Design review of the part built by this model. Coordinates are the model's own, in mm. Face numbers are marked on the shaded views. Coordinates: 2 decimals unless noted, no trailing zeros. Loops run counter-clockwise (first coordinate to the right, second up) from the corner with the lowest first, then second, coordinate; pieces in that order, holes last. Notation, with made-up numbers: M 71.25,78.25 L 118.25,78.25 A15 cw 118.25,98.25 Z; hole C 51,-27 d10. An arc over 180 degrees is marked long. Answer as CSV lines item,"result". Start each with the question number.
from build123d import *

# Parameters (mm, degrees)
F1_DEPTH = 100
F2_R     = 2
F2_R_2   = 1
F3_DEPTH = 14.501


with BuildPart() as f1:
    # F0 (on Right) → F1 (new body)
    with BuildSketch(Plane.YZ):
        with BuildLine():
            ThreePointArc((10, 8.5), (9.56066, 9.56066), (8.5, 10))
            Line((8.5, 10), (3, 10))
            Line((3, 10), (3, 8.5))
            Line((3, 8.5), (6, 8.5))
            Line((6, 8.5), (6, 7))
            Line((6, 7), (3.75, 4.5))
            Line((3.75, 4.5), (0, 4.5))
            Line((0, 4.5), (-3.75, 4.5))
            Line((-3.75, 4.5), (-6, 7))
            Line((-6, 7), (-6, 8.5))
            Line((-6, 8.5), (-3, 8.5))
            Line((-3, 8.5), (-3, 10))
            Line((-3, 10), (-8.5, 10))
            ThreePointArc((-8.5, 10), (-9.56066, 9.56066), (-10, 8.5))
            Line((-10, 8.5), (-10, 3))
            Line((-10, 3), (-8.5, 3))
            Line((-8.5, 3), (-8.5, 6))
            Line((-8.5, 6), (-7, 6))
            Line((-7, 6), (-4.5, 3.75))
            Line((-4.5, 3.75), (-4.5, 0))
            Line((-4.5, 0), (-4.5, -3.75))
            Line((-4.5, -3.75), (-7, -6))
            Line((-7, -6), (-8.5, -6))
            Line((-8.5, -6), (-8.5, -3))
            Line((-8.5, -3), (-10, -3))
            Line((-10, -3), (-10, -8.5))
            ThreePointArc((-10, -8.5), (-9.56066, -9.56066), (-8.5, -10))
            Line((-8.5, -10), (-3, -10))
            Line((-3, -10), (-3, -8.5))
            Line((-3, -8.5), (-6, -8.5))
            Line((-6, -8.5), (-6, -7))
            Line((-6, -7), (-3.75, -4.5))
            Line((-3.75, -4.5), (0, -4.5))
            Line((0, -4.5), (3.75, -4.5))
            Line((3.75, -4.5), (6, -7))
            Line((6, -7), (6, -8.5))
            Line((6, -8.5), (3, -8.5))
            Line((3, -8.5), (3, -10))
            Line((3, -10), (8.5, -10))
            ThreePointArc((8.5, -10), (9.56066, -9.56066), (10, -8.5))
            Line((10, -8.5), (10, -3))
            Line((10, -3), (8.5, -3))
            Line((8.5, -3), (8.5, -6))
            Line((8.5, -6), (7, -6))
            Line((7, -6), (4.5, -3.75))
            Line((4.5, -3.75), (4.5, 0))
            Line((4.5, 0), (4.5, 3.75))
            Line((4.5, 3.75), (7, 6))
            Line((7, 6), (8.5, 6))
            Line((8.5, 6), (8.5, 3))
            Line((8.5, 3), (10, 3))
            Line((10, 3), (10, 8.5))
        make_face()
    extrude(amount=F1_DEPTH)

    # F2 (on face) → F3 (cut, through all)
    with BuildSketch(Plane.XY.offset(4.5)):
        with Locations((86, 0)):
            Circle(F2_R)
        with Locations((95, 0)):
            Circle(F2_R)
        with Locations((40, 0)):
            Circle(F2_R_2)
    extrude(amount=-F3_DEPTH, mode=Mode.SUBTRACT)


solid = f1.part
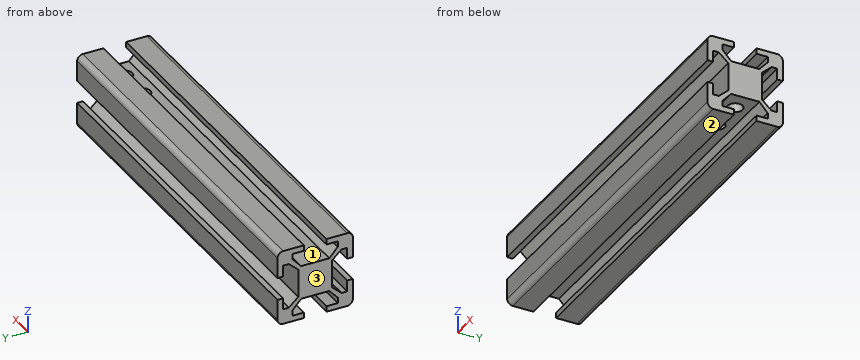
Item 1: Mouldability with a two-part tool opening along Z and no side actions: class the marked faces 1, 2 and 3 as released by +Z, released by -Z, zero draft, split by the parting line, or undercut.
Item 2: For pin 1 (1 mm diameter, centred on x = 55, z = -2, fed in from +Y); pin 2 (1.2 mm diameter, centred on x = 46.5, y = 9.5, fed in from -Z); pin 3 (0.8 mm diameter, centred on x = 52.5, y = 9, fed in from +Z); pin 4 (2 mm diameter, centred on y = 7, z = 1.5, fed in from -X), all flat-tipped, find the tip position at first contact; note any pin that passes through.
Item 3: Add section A-A (y = 0). Give the boundary of the cut face in (x, z), plus the area to 3 significant figures.
Item 4: For line 1 along Z through (x, y) = (95, -3.25); line 2 along Z through (x, y) = (50, -8.25); line 3 along Y through (x, z) = (95, 1.25), list the stretches that pass through material, from the lowest coordinate up. Write a range as from..to.
Response:
1,face 1,"undercut"
1,face 2,"released by -Z"
1,face 3,"zero draft"
2,pin 1,"y = 4.5"
2,pin 2,"z = -9.95"
2,pin 3,"z = 10"
2,pin 4,"through"
3,outline,"M 0,-4.5 L 39,-4.5 L 39,4.5 L 0,4.5 Z; M 41,-4.5 L 84,-4.5 L 84,4.5 L 41,4.5 Z; M 88,-4.5 L 93,-4.5 L 93,4.5 L 88,4.5 Z; M 97,-4.5 L 100,-4.5 L 100,4.5 L 97,4.5 Z"
3,area,"810 mm²"
4,line 1,"-10..-8.5, -4.5..4.5, 8.5..10"
4,line 2,"-10..-6, 6..10"
4,line 3,"-4.5..-2, 2..4.5"
